For this review, use the dimensioned drawing (mm, ordinates from the lowest corner) and the shaded views. A direction names the side the tool comes from. Coordinates: 2 decimals unless noted, no trailing zeros. Write each loop counter-clockwise with the first axis right and the second up, starting at its lowest first coordinate (ties: lowest second). Pieces come first, ordered by that corner, then holes. Notation, with made-up numbers: (69.25, 86) -> (90.25, 86) arc R16 ccw to (90.25, 92) -> close; hole circle Ø7 at (-1, 85.25). An arc over 180 degrees is marked (long way). Put each result on its own line as item: value. Start each with the question number.
Item 1: Insertion check: P1, Ø8, axis at x = 8, z = 64, coming from the +Y side (1 decimal); P2, Ø7, axis at x = 35.5, y = 16.5, coming from the -Z side; P3, Ø4, axis at y = 15.5, z = 53, coming from the +X side (1 decimal); P4, Ø11, axis at x = 30.5, z = 36, coming from the +Y side. Each pin has a flat end and moves straight along its axis. Give the tip position at first contact, or say it passes through.
Item 2: To check wall thickness, follow L1, parallel to X at y = 17, z = 38.5; L2, parallel to Y at x = 59.5, z = 62.5 (1 decimal); L3, parallel to X at y = 17.25, z = 44 (1 decimal). State the ranges of each line that lie inside material, in increasing order.
Item 3: The part is to be moulded in two halves that separate along Z. For the marked faces 1, 2 and 3, say which applies: +Z half, -Z half, draft (parallel to the pull), parting line (faces both ways), or undercut.
Item 4: Consider section C-C on y = 16.5. Give the boundary of the cut face in (x, z) (1 decimal).
Item 5: For the marked faces 4, 5, 6 and 7, list the 3-axis set-ups (+Z, -Z, +X, -X, +Y, -Y) from which the entire face can be reached by the end or side of a thin tool; tool diameter is ignored.
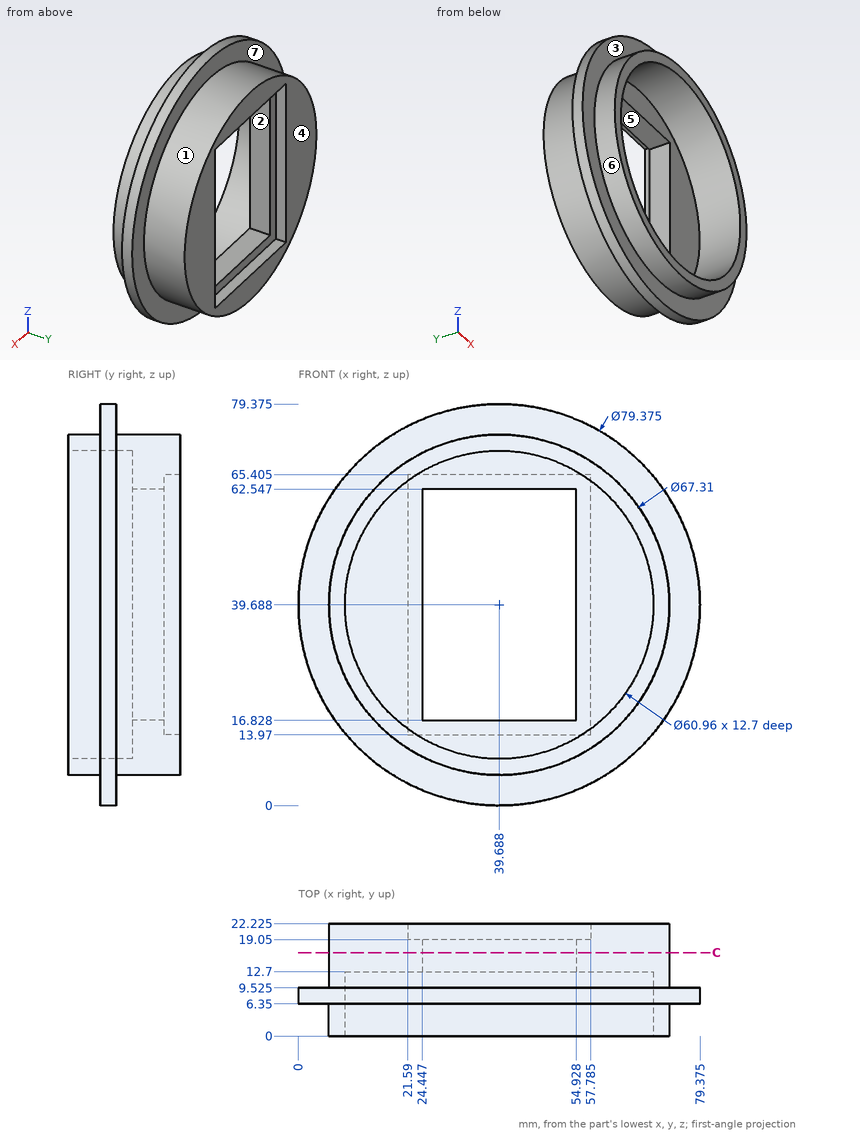
Return value:
1. P1: y = 9.5
1. P2: z = 6.04
1. P3: x = 71.4
1. P4: through
2. L1: 6.05 to 24.45, 54.93 to 73.32
2. L2: 12.7 to 22.2
2. L3: 6.3 to 24.4, 54.9 to 73.1
3. face 1: parting line
3. face 2: undercut
3. face 3: draft
4. outline: circle Ø67.3 at (39.7, 39.7); hole (24.4, 16.8) -> (54.9, 16.8) -> (54.9, 62.5) -> (24.4, 62.5) -> close
5. face 4: +Z, -Z, +X, -X, +Y
5. face 5: +Y, -Y
5. face 6: -Y
5. face 7: +Y
